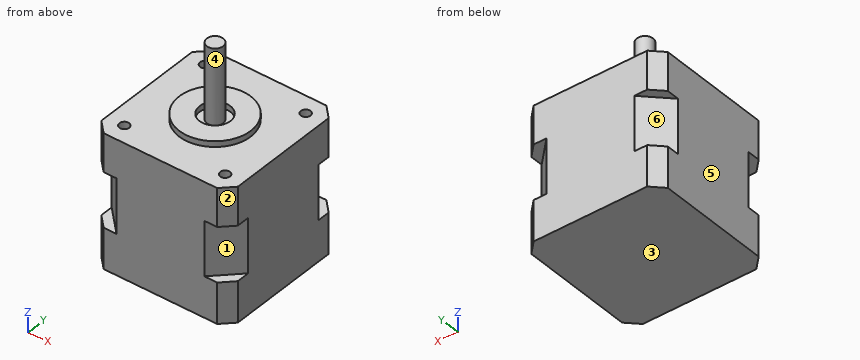
from build123d import *

# Parameters (mm, degrees)
F1_DEPTH  = 12.5
F3_DEPTH  = 16.75
F4_START  = 29.25
F4_DEPTH  = 11.75
F5_R      = 1.5
F6_DEPTH  = 5.5
F7_R      = 11
F7_R_2    = 4.75
F8_DEPTH  = 1.75
F9_R      = 2.5
F10_DEPTH = 23.25


with BuildPart() as f1:
    # F0 (on Top) → F1 (new body)
    with BuildSketch(Plane.XY):
        Polygon((17.4644660941, 21), (-17.4644660941, 21), (-21, 17.4644660941), (-21, -17.4644660941), (-17.4644660941, -21), (17.4644660941, -21), (21, -17.4644660941), (21, 17.4644660941), align=None)
    extrude(amount=F1_DEPTH)

    # F2 (on face) → F3 (join)
    with BuildSketch(Plane.XY.offset(12.5)):
        Polygon((13.5000012147, 21), (-13.4999987853, 21), (-21, 13.4999987853), (-21, -13.5000012147), (-13.5000012147, -21), (13.4999987853, -21), (21, -13.4999987853), (21, 13.5000012147), align=None)
    extrude(amount=F3_DEPTH)

    # F0 (on Top) → F4 (join)
    with BuildSketch(Plane.XY.offset(F4_START)):
        Polygon((17.4644660941, 21), (-17.4644660941, 21), (-21, 17.4644660941), (-21, -17.4644660941), (-17.4644660941, -21), (17.4644660941, -21), (21, -17.4644660941), (21, 17.4644660941), align=None)
    extrude(amount=F4_DEPTH)

    # F5 (on face) → F6 (cut)
    with BuildSketch(Plane.XY.offset(41)):
        with Locations((-15.5, 15.5)):
            Circle(F5_R)
        with Locations((15.5, 15.5)):
            Circle(F5_R)
        with Locations((15.5, -15.5)):
            Circle(F5_R)
        with Locations((-15.5, -15.5)):
            Circle(F5_R)
    extrude(amount=-F6_DEPTH, mode=Mode.SUBTRACT)

    # F7 (on face) → F8 (join)
    with BuildSketch(Plane.XY.offset(41)):
        Circle(F7_R)
        Circle(F7_R_2, mode=Mode.SUBTRACT)
    extrude(amount=F8_DEPTH)

    # F9 (on face) → F10 (join)
    with BuildSketch(Plane.XY.offset(41)):
        Circle(F9_R)
    extrude(amount=F10_DEPTH)


solid = f1.part
Geometry check sheet. Reference: the model listing, model coordinates, mm. Face numbers are marked on the shaded views. A direction names the side the tool comes from. Round coordinates to 2 decimals unless told otherwise and drop trailing zeros. Loops run counter-clockwise (first coordinate to the right, second up) from the corner with the lowest first, then second, coordinate; pieces in that order, holes last.
Item 1: Thickness scan on line 1 (Y direction, x = -15.5, z = 37.1); line 2 (Z direction, x = -19, y = -17); line 3 (Z direction, x = 10, y = 6.5). Record the ranges inside material, lowest first.
Item 2: Gauge pin test, flat ends, axial feed: pin 1 (3.5 mm diameter, centred on x = -15, y = 15.5, fed in from +Z); pin 2 (17.5 mm diameter, centred on x = -4, y = 1.5, fed in from +Z); pin 3 (1.5 mm diameter, centred on x = 15, y = -15.5, fed in from +Z); pin 4 (10 mm diameter, centred on y = 7, z = 51, fed in from +X). Record the tip position at first contact, or that the pin passes through.
Item 3: Cross-section at A-A on y = 0. Record the boundary of the cut face in (x, z), then the cut area to 3 significant figures.
Item 4: Cross-section at B-B on x = 15.5. Record the boundary of the cut face in (y, z), then the cut area to 3 significant figures.
Item 5: Mould release check, pull along Z, two halves, no side actions. Record for the marked faces 1, 2 and 3: pulls with the +Z half, pulls with the -Z half, needs draft (parallel to the pull), parting line crosses it, or undercut.
Item 6: Cross-section at C-C on z = 28. Record the boundary of the cut face in (x, y).
Item 7: Access from +Z, -Z, +X, -X, +Y, -Y to the whole of each face (thin tool, end or side, straight path). Record for the marked faces 4, 5 and 6.
Answer sheet:
1. line 1: y = -21 to -17, -14 to 14, 17 to 21
1. line 2: z = 0 to 12.5, 29.25 to 41
1. line 3: z = 0 to 41
2. pin 1: stops at z = 41
2. pin 2: stops at z = 64.25
2. pin 3: stops at z = 35.5
2. pin 4: stops at x = 1.5
3. outline: (-21, 0) - (21, 0) - (21, 41) - (11, 41) - (11, 42.75) - (4.75, 42.75) - (4.75, 41) - (2.5, 41) - (2.5, 64.25) - (-2.5, 64.25) - (-2.5, 41) - (-4.75, 41) - (-4.75, 42.75) - (-11, 42.75) - (-11, 41) - (-21, 41) - close
3. area: 1,860 mm2
4. outline: (-21, 0) - (21, 0) - (21, 12.5) - (19, 12.5) - (19, 29.25) - (21, 29.25) - (21, 41) - (17, 41) - (17, 35.5) - (14, 35.5) - (14, 41) - (-14, 41) - (-14, 35.5) - (-17, 35.5) - (-17, 41) - (-21, 41) - (-21, 29.25) - (-19, 29.25) - (-19, 12.5) - (-21, 12.5) - close
4. area: 1,620 mm2
5. face 1: undercut
5. face 2: needs draft
5. face 3: pulls with the -Z half
6. outline: (-21, -13.5) - (-13.5, -21) - (13.5, -21) - (21, -13.5) - (21, 13.5) - (13.5, 21) - (-13.5, 21) - (-21, 13.5) - close
7. face 4: +Z
7. face 5: +Z, -Z, -X, +Y, -Y
7. face 6: -X, +Y
